from build123d import *

# Parameters (mm, degrees)
EXTRUDE_1_DEPTH     = 30
SKETCH_2_W          = 20
SKETCH_2_H          = 2
EXTRUDE_2_DEPTH     = 6
SKETCH_3_W          = 10
SKETCH_3_H          = 10
EXTRUDE_5_DEPTH     = 10
SKETCH_3_2_W        = 10
SKETCH_3_2_H        = 10
CUT_EXTRUDE_1_DEPTH = 8
SKETCH_4_R          = 1
CUT_EXTRUDE_2_DEPTH = 15


with BuildPart() as part:
    # 草图1 → 凸台-拉伸1 (new body)
    with BuildSketch(Plane(origin=(0, 0, 0), x_dir=(1, 0, 0), z_dir=(0, 1, 0))):
        Polygon((-38.526315789, 0), (5.473684211, 0), (5.473684211, 10), (7.436715789, 10), (7.436715789, -2), (5.473684211, -2), (-38.526315789, -2), (-40.526315789, -2), (-40.526315789, 10), (-38.526315789, 10), align=None)
    extrude(amount=EXTRUDE_1_DEPTH)

    # 草图2 → 凸台-拉伸2 (add)
    with BuildSketch(Plane.XY):
        with Locations((-16.563284211, 1)):
            Rectangle(SKETCH_2_W, SKETCH_2_H)
    extrude(amount=-EXTRUDE_2_DEPTH)

    # 草图3 → 凸台-拉伸5 (add)
    with BuildSketch(Plane.XY):
        with Locations((-45.526315789, 5)):
            Rectangle(SKETCH_3_W, SKETCH_3_H)
        with Locations((12.436715789, 5)):
            Rectangle(SKETCH_3_W, SKETCH_3_H)
    extrude(amount=-EXTRUDE_5_DEPTH)

    # 草图3<2> → 切除-拉伸1 (cut)
    with BuildSketch(Plane.XY):
        with Locations((-45.526315789, 5)):
            Rectangle(SKETCH_3_2_W, SKETCH_3_2_H)
        with Locations((12.436715789, 5)):
            Rectangle(SKETCH_3_2_W, SKETCH_3_2_H)
    extrude(amount=-CUT_EXTRUDE_1_DEPTH, mode=Mode.SUBTRACT)

    # 草图4 → 切除-拉伸2 (cut)
    with BuildSketch(Plane.XY):
        with Locations((-45.867673878, 4.706880403)):
            Circle(SKETCH_4_R)
        with Locations((12.075128271, 4.706880403)):
            Circle(SKETCH_4_R)
    extrude(amount=-CUT_EXTRUDE_2_DEPTH, mode=Mode.SUBTRACT)


solid = part.part
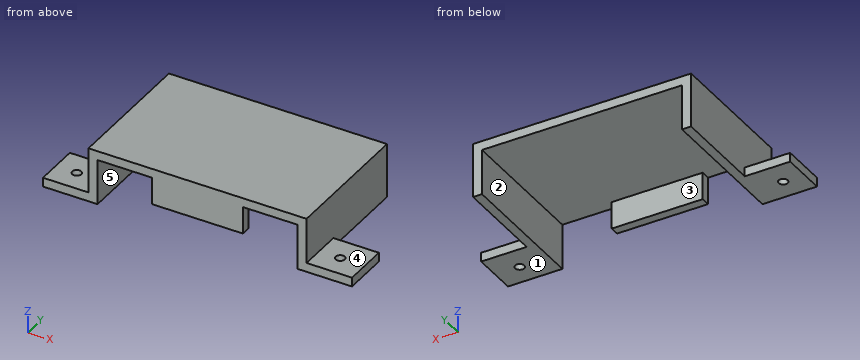
Verification items for the finished model (mm, model axes). Face numbers are marked on the shaded views. A direction names the side the tool comes from. Coordinates: 2 decimals unless noted, no trailing zeros. Order: outer loops, then holes, each group sorted by start corner. A loop starts at its lowest first (then second) coordinate and runs counter-clockwise, first axis right, second up. Notation, with made-up numbers: M -20.75,73.25 L -8.75,73.25 A21 cw -8.75,79.25 Z; hole C 68.5,88 d6. An arc over 180 degrees is marked long. One line per item, written item: value. Start each with the question number.
Item 1: Scan lines: probe 1 along X at (y, z) = (1.5, -4.75); probe 2 along X at (y, z) = (26, -3.25); probe 3 along X at (y, z) = (4.5, -9.5). Record each from-to range of solid material in increasing order.
Item 2: Access from +Z, -Z, +X, -X, +Y, -Y to the whole of each face (thin tool, end or side, straight path). Record for the marked faces 3, 4 and 5.
Item 3: Mould release check, pull along X, two halves, no side actions. Record for the marked faces 1 and 2: released by +X, released by -X, zero draft, split by the parting line, or undercut.
Item 4: Sectioned sample at A-A (z = -7.25). Enter the section's corners in (x, y), then the cut area to 3 significant figures.
Item 5: Sectioned sample at D-D (y = 21). Enter the section's corners in (x, z).
Item 6: Gauge pin test, flat ends, axial feed: pin 1 (0.6 mm diameter, centred on x = -45.5, z = -9, fed in from +Y); pin 2 (1.5 mm diameter, centred on x = -20, z = -3.5, fed in from +Y); pin 3 (1 mm diameter, centred on x = -15, y = 1, fed in from -Z); pin 4 (5 mm diameter, centred on x = -3, z = -4.5, fed in from -Y) (1 decimal). Record the tip position at first contact, or that the pin passes through.
Item 7: Sectioned sample at B-B (x = -46). Enter the section's corners in (y, z).
Item 8: Sectioned sample at C-C (z = -1.5). Enter the section's corners in (x, y).
Conclusion:
1. probe 1: x = -40.53 to -38.53, -26.56 to -6.56, 5.47 to 7.44
1. probe 2: x = -40.53 to -38.53, 5.47 to 7.44
1. probe 3: x = -50.53 to -46.85, -44.89 to -38.53, 5.47 to 11.1, 13.05 to 17.44
2. face 3: -Z, +Y
2. face 4: +Z, +X, +Y, -Y
2. face 5: -Z, +Y, -Y
3. face 1: zero draft
3. face 2: undercut
4. outline: M -40.53,0 L -38.53,0 L -38.53,30 L -40.53,30 Z; M 5.47,0 L 7.44,0 L 7.44,30 L 5.47,30 Z
4. area: 119 mm^2
5. outline: M -40.53,-10 L -38.53,-10 L -38.53,0 L 5.47,0 L 5.47,-10 L 7.44,-10 L 7.44,2 L -40.53,2 Z
6. pin 1: stops at y = 10
6. pin 2: stops at y = 2
6. pin 3: stops at z = -6
6. pin 4: passes through
7. outline: M 0,-10 L 3.72,-10 L 3.72,-8 L 0,-8 Z; M 5.7,-10 L 10,-10 L 10,-8 L 5.7,-8 Z
8. outline: M -40.53,0 L -38.53,0 L -38.53,30 L -40.53,30 Z; M -26.56,0 L -6.56,0 L -6.56,2 L -26.56,2 Z; M 5.47,0 L 7.44,0 L 7.44,30 L 5.47,30 Z
